```python
from build123d import *

# Parameters (mm, degrees)
SKETCH1_R           = 3.025
BOSS_EXTRUDE1_DEPTH = 56.6


with BuildPart() as part:
    # Sketch1 → Boss-Extrude1 (new body)
    with BuildSketch(Plane(origin=(0, 0, 0), x_dir=(1, 0, 0), z_dir=(0, 1, 0))):
        with BuildLine():
            Line((-6, 0), (-6, 5.43))
            Line((-6, 5.43), (-6, 6))
            Line((-6, 6), (6, 6))
            Line((6, 6), (6, 5.43))
            Line((6, 5.43), (6, 0))
            ThreePointArc((6, 0), (0, -6), (-6, 0))
        make_face()
        Circle(SKETCH1_R, mode=Mode.SUBTRACT)
    extrude(amount=BOSS_EXTRUDE1_DEPTH)


solid = part.part
```
Geometry: final body of the model. Coordinates: model frame, mm. Round coordinates to 2 decimals unless told otherwise and drop trailing zeros. Write each loop counter-clockwise with the first axis right and the second up, starting at its lowest first coordinate (ties: lowest second). Pieces come first, ordered by that corner, then holes. Notation, with made-up numbers: M -18.5,5 L 15.5,5 A19 cw 15.5,37 Z; hole C 70.5,-11.75 d6. An arc over 180 degrees is marked long. Answer in a Markdown table with one row per item. Add a question column.
(1) Draft query along X for faces 1 (the face through (-6, 28, -3)), 2 (the face through (2.794, 27.904, 1.159)), 3 (the face through (6, 28, -3)). Return one class per face: pulls with the +X half, pulls with the -X half, needs draft (parallel to the pull), parting line crosses it, or undercut.
(2) Contact query for flat-ended pins moving along their axis: pin 1 (4 mm diameter, centred on y = 33.5, z = 3.5, fed in from +X); pin 2 (4 mm diameter, centred on y = 38, z = 4.5, fed in from -X). Output: stop coordinate, or through.
(3) Ray query, L1, parallel to X at y = 31, z = 0 (3 decimals); L2, parallel to Z at x = 1, y = 28. Return the intervals inside material, ascending.
(4) Cut plane D-D, the plane x = 3.5. Return the cut outline in (y, z).
(5) Cut plane B-B, the plane y = 45.5. Return the cut outline in (x, z) (3 decimals), then the cut area to 3 significant figures.
(6) Cut plane A-A, the plane x = 0. Return the cut outline in (y, z) (3 decimals).
(7) Cut plane C-C, the plane z = 1.25. Return the cut outline in (x, y).
Established:
| question | item | result |
|---|---|---|
| 1 | face 1 | pulls with the -X half |
| 1 | face 2 | undercut |
| 1 | face 3 | pulls with the +X half |
| 2 | pin 1 | x = 5.81 |
| 2 | pin 2 | x = -5.45 |
| 3 | L1 | -6 to -3.025, 3.025 to 6 |
| 3 | L2 | -6 to -2.85, 2.85 to 5.92 |
| 4 | outline | M 0,-6 L 56.6,-6 L 56.6,4.87 L 0,4.87 Z |
| 5 | outline | M -6,-6 L 6,-6 L 6,0 A6 ccw -6,0 Z; hole C 0,0 d6.05 |
| 5 | area | 99.8 mm² |
| 6 | outline | M 0,-6 L 56.6,-6 L 56.6,-3.025 L 0,-3.025 Z; M 0,3.025 L 56.6,3.025 L 56.6,6 L 0,6 Z |
| 7 | outline | M -5.87,0 L -2.75,0 L -2.75,56.6 L -5.87,56.6 Z; M 2.75,0 L 5.87,0 L 5.87,56.6 L 2.75,56.6 Z |
